from build123d import *

# Parameters (mm, degrees)
BOSS_EXTRUDE1_DEPTH  = 6
EXTRUDE_THIN1_DEPTH  = 20
SKETCH3_R            = 2.75
CUT_EXTRUDE1_DEPTH   = 1.5
LPATTERN1_COUNT      = 4
LPATTERN1_PITCH      = 30
LPATTERN1_COUNT_DIR2 = 4
LPATTERN1_PITCH_DIR2 = 30
FILLET1_R            = 4
SKETCH4_R            = 1.5
BOSS_EXTRUDE2_DEPTH  = 50
SKETCH5_R            = 1.65
CUT_EXTRUDE2_DEPTH   = 51
SKETCH6_R            = 1
CUT_EXTRUDE3_DEPTH   = 107.809409698
LPATTERN2_COUNT      = 4
LPATTERN2_PITCH      = 30
SKETCH7_R            = 1
CUT_EXTRUDE4_DEPTH   = 107.809409698
LPATTERN3_COUNT      = 4
LPATTERN3_PITCH      = 30


with BuildPart() as part:
    # Sketch1 → Boss-Extrude1 (new body)
    with BuildSketch(Plane(origin=(0, 0, 0), x_dir=(1, 0, 0), z_dir=(0, 1, 0))):
        with BuildLine():
            Line((-56.5, 72.5), (72.5, 72.5))
            Line((72.5, 72.5), (72.5, -72.5))
            Line((72.5, -72.5), (-72.5, -72.5))
            Line((-72.5, -72.5), (-72.5, 56.5))
            ThreePointArc((-72.5, 56.5), (-67.813708499, 67.813708499), (-56.5, 72.5))
        make_face()
    extrude(amount=BOSS_EXTRUDE1_DEPTH)

    # Sketch2 → Extrude-Thin1 (add)
    with BuildSketch(Plane(origin=(0, 6, 0), x_dir=(1, 0, 0), z_dir=(0, 1, 0))):
        with BuildLine():
            Line((-72.5, -72.5), (-72.5, 56.5))
            ThreePointArc((-72.5, 56.5), (-67.813708499, 67.813708499), (-56.5, 72.5))
            Line((-56.5, 72.5), (72.5, 72.5))
            Line((72.5, 72.5), (72.5, 62.5))
            Line((72.5, 62.5), (-56.5, 62.5))
            ThreePointArc((-56.5, 62.5), (-60.742640687, 60.742640687), (-62.5, 56.5))
            Line((-62.5, 56.5), (-62.5, -72.5))
            Line((-62.5, -72.5), (-72.5, -72.5))
        make_face()
    extrude(amount=EXTRUDE_THIN1_DEPTH)

    # Sketch3 → Cut-Extrude1 (cut)
    with BuildSketch(Plane(origin=(0, 6, 0), x_dir=(1, 0, 0), z_dir=(0, 1, 0))):
        with Locations(Location((57.5, -57.5, 0), (0, 0, 270))):
            Circle(SKETCH3_R)
    cut_extrude1 = extrude(amount=-CUT_EXTRUDE1_DEPTH, mode=Mode.SUBTRACT)

    # LPattern1: Cut-Extrude1 4 × 4
    with Locations(*[(-i * LPATTERN1_PITCH, 0, -j * LPATTERN1_PITCH_DIR2) for i in range(LPATTERN1_COUNT) for j in range(LPATTERN1_COUNT_DIR2) if (i, j) != (0, 0)]):
        add(cut_extrude1, mode=Mode.SUBTRACT)

    # Fillet1
    fillet1_edges = [part.edges().sort_by_distance(p)[0] for p in [
        (8, 26, -72.5),
        (-67.813708499, 26, -67.813708499),
        (-72.5, 26, 8),
        (8, 26, -62.5),
        (-62.5, 26, 8),
        (-60.742640687, 26, -60.742640687),
    ]]
    fillet(fillet1_edges, radius=FILLET1_R)

    # Sketch4 → Boss-Extrude2 (add, symmetric)
    with BuildSketch(Plane(origin=(0, 0, 0), x_dir=(0, 0, -1), z_dir=(1, 0, 0))):
        with Locations((-72.5, 3)):
            Circle(SKETCH4_R)
    extrude(amount=BOSS_EXTRUDE2_DEPTH, both=True)

    # Sketch5 → Cut-Extrude2 (cut, symmetric)
    with BuildSketch(Plane.XY):
        with Locations((72.5, 3)):
            Circle(SKETCH5_R)
    extrude(amount=CUT_EXTRUDE2_DEPTH, both=True, mode=Mode.SUBTRACT)

    # Sketch6 → Cut-Extrude3 (cut, symmetric)
    with BuildSketch(Plane.XY):
        with Locations((-50, 0)):
            Circle(SKETCH6_R)
    cut_extrude3 = extrude(amount=CUT_EXTRUDE3_DEPTH, both=True, mode=Mode.SUBTRACT)

    # LPattern2: Cut-Extrude3 ×4
    with Locations(*[(i * LPATTERN2_PITCH, 0, 0) for i in range(1, LPATTERN2_COUNT)]):
        add(cut_extrude3, mode=Mode.SUBTRACT)

    # Sketch7 → Cut-Extrude4 (cut, symmetric)
    with BuildSketch(Plane(origin=(0, 0, 0), x_dir=(0, 0, -1), z_dir=(1, 0, 0))):
        with Locations((50, 0)):
            Circle(SKETCH7_R)
    cut_extrude4 = extrude(amount=CUT_EXTRUDE4_DEPTH, both=True, mode=Mode.SUBTRACT)

    # LPattern3: Cut-Extrude4 ×4
    with Locations(*[(0, 0, i * LPATTERN3_PITCH) for i in range(1, LPATTERN3_COUNT)]):
        add(cut_extrude4, mode=Mode.SUBTRACT)


solid = part.part
The listing builds one solid part. Answer for the finished solid, in the listing's coordinates (mm). A direction names the side the tool comes from. Round coordinates to 2 decimals unless told otherwise and drop trailing zeros. Order: outer loops, then holes, each group sorted by start corner. A loop starts at its lowest first (then second) coordinate and runs counter-clockwise, first axis right, second up. Notation, with made-up numbers: (84, 48.5) -> (133, 48.5) arc R17 ccw to (133, 65.5) -> close; hole circle Ø3 at (6.25, -38.75). An arc over 180 degrees is marked (long way). Write each question's results on one line, items separated by ' | '. Start each with the question number.
Q1. Each of these flat-tipped pins is pushed along its axis until it touches: pin 1 (1.5 mm diameter, centred on x = 39.5, y = 4.5, fed in from +Z); pin 2 (5 mm diameter, centred on y = 10.5, z = -17.5, fed in from +X); pin 3 (4.5 mm diameter, centred on x = -33.5, z = 56.5, fed in from +Y). Where does it stop, or does it pass through?
Q2. Find section A-A (z = -42). Determine the outline of the cut face in (x, y).
Q3. The mould has two halves that part along X. Classify faces 1 (the flat face through (-62, 0, 25)), 2 (the cylindrical face through (-63.703, 24.859, 8.903)), 3 (the flat face through (-32, 4.5, 27)): pulls with the +X half, pulls with the -X half, needs draft (parallel to the pull), parting line crosses it, or undercut.
Q4. Straight lines are drawn through the part: probe 1 along X at (y, z) = (5.05, -32.5); probe 2 along Y at (x, z) = (40, 14); probe 3 along Z at (x, y) = (17, 6.25). For each, find the intervals that lie inside material, in ascending order. Write a range as from..to.
Q5. Which of the six approach directions +Z, -Z, +X, -X, +Y, -Y give full straight-line access (tool end or side, diameter ignored) to faces 4 (the flat face through (-62.5, 14, 7)), 5 (the cylindrical face through (-71.297, 24.859, 7.097)), 6 (the flat face through (-2, 4.5, -33))?
Q6. Find section B-B (x = 32). Determine the outline of the cut face in (y, z), then the cut area to 3 significant figures.
Q7. Find section C-C (y = 14). Determine the outline of the cut face in (x, z).
Worked answers:
1) pin 1: stops at z = 73.8 | pin 2: stops at x = -62.5 | pin 3: stops at y = 6
2) outline: (-72.5, 0) -> (-51, 0) arc R1 cw to (-49, 0) -> (-21, 0) arc R1 cw to (-19, 0) -> (9, 0) arc R1 cw to (11, 0) -> (39, 0) arc R1 cw to (41, 0) -> (72.5, 0) -> (72.5, 1.35) arc R1.65 cw to (72.5, 4.65) -> (72.5, 6) -> (-62.5, 6) -> (-62.5, 22) arc R4 ccw to (-66.5, 26) -> (-68.5, 26) arc R4 ccw to (-72.5, 22) -> close
3) face 1: needs draft | face 2: pulls with the +X half | face 3: undercut
4) probe 1: x = -72.5..-35.25, -29.75..-5.25, 0.25..24.75, 30.25..54.75, 60.25..72.5 | probe 2: y = 1..6 | probe 3: z = -72.5..-62.5
5) face 4: +Z, +X, +Y | face 5: +Z, -Z, -X, +Y | face 6: +Y
6) outline: (0, -72.5) -> (22, -72.5) arc R4 ccw to (26, -68.5) -> (26, -66.5) arc R4 ccw to (22, -62.5) -> (6, -62.5) -> (6, 72.5) -> (4.5, 72.5) arc R1.5 ccw to (1.5, 72.5) -> (0, 72.5) -> (0, 41) arc R1 cw to (0, 39) -> (0, 11) arc R1 cw to (0, 9) -> (0, -19) arc R1 cw to (0, -21) -> (0, -49) arc R1 cw to (0, -51) -> close | area: 1,060 mm2
7) outline: (-72.5, -56.5) arc R16 ccw to (-56.5, -72.5) -> (72.5, -72.5) -> (72.5, -62.5) -> (-56.5, -62.5) arc R6 cw to (-62.5, -56.5) -> (-62.5, 72.5) -> (-72.5, 72.5) -> close
